```python
from build123d import *

# Parameters (mm, degrees)
BOSS_EXTRU_1_DEPTH         = 3
ESQUISSE2_W                = 10
ESQUISSE2_H                = 3
ENL_V_MAT_EXTRU_1_DEPTH    = 3
R_P_TITION_LIN_AIRE1_COUNT = 8
R_P_TITION_LIN_AIRE1_PITCH = 20
ESQUISSE4_W                = 3
ESQUISSE4_H                = 10
BOSS_EXTRU_2_DEPTH         = 3
R_P_TITION_LIN_AIRE3_COUNT = 2
R_P_TITION_LIN_AIRE3_PITCH = 20
ESQUISSE5_W                = 10
ESQUISSE5_H                = 3
ENL_V_MAT_EXTRU_3_DEPTH    = 3
R_P_TITION_LIN_AIRE4_COUNT = 4
R_P_TITION_LIN_AIRE4_PITCH = 20
ESQUISSE6_W                = 10
ESQUISSE6_H                = 3
ENL_V_MAT_EXTRU_4_DEPTH    = 3
R_P_TITION_LIN_AIRE5_COUNT = 3
R_P_TITION_LIN_AIRE5_PITCH = 20
ESQUISSE7_W                = 3
ESQUISSE7_H                = 10
ENL_V_MAT_EXTRU_5_DEPTH    = 3
R_P_TITION_LIN_AIRE6_COUNT = 3
R_P_TITION_LIN_AIRE6_PITCH = 20


with BuildPart() as part:
    # Esquisse1 → Boss.-Extru.1 (new body)
    with BuildSketch(Plane.XY):
        Polygon((163, 0), (163, -110), (113, -110), (113, -43), (0, -43), (0, 0), align=None)
    extrude(amount=BOSS_EXTRU_1_DEPTH)

    # Esquisse2 → Enlèv. mat.-Extru.1 (cut)
    with BuildSketch(Plane.XY.offset(3)):
        with Locations((5, -1.5)):
            Rectangle(ESQUISSE2_W, ESQUISSE2_H)
    enl_v_mat_extru_1 = extrude(amount=-ENL_V_MAT_EXTRU_1_DEPTH, mode=Mode.SUBTRACT)

    # Répétition linéaire1: Enlèv. mat.-Extru.1 ×8
    with Locations(*[(i * R_P_TITION_LIN_AIRE1_PITCH, 0, 0) for i in range(1, R_P_TITION_LIN_AIRE1_COUNT)]):
        add(enl_v_mat_extru_1, mode=Mode.SUBTRACT)

    # Esquisse4 → Boss.-Extru.2 (add)
    with BuildSketch(Plane.ZY):
        with Locations((1.5, -38)):
            Rectangle(ESQUISSE4_W, ESQUISSE4_H)
    boss_extru_2 = extrude(amount=BOSS_EXTRU_2_DEPTH)

    # Répétition linéaire3: Boss.-Extru.2 ×2
    with Locations(*[(0, i * R_P_TITION_LIN_AIRE3_PITCH, 0) for i in range(1, R_P_TITION_LIN_AIRE3_COUNT)]):
        add(boss_extru_2)

    # Esquisse5 → Enlèv. mat.-Extru.3 (cut)
    with BuildSketch(Plane.XY.offset(3)):
        with Locations((108, -41.5)):
            Rectangle(ESQUISSE5_W, ESQUISSE5_H)
    enl_v_mat_extru_3 = extrude(amount=-ENL_V_MAT_EXTRU_3_DEPTH, mode=Mode.SUBTRACT)

    # Répétition linéaire4: Enlèv. mat.-Extru.3 ×4
    with Locations(*[(-i * R_P_TITION_LIN_AIRE4_PITCH, 0, 0) for i in range(1, R_P_TITION_LIN_AIRE4_COUNT)]):
        add(enl_v_mat_extru_3, mode=Mode.SUBTRACT)

    # Esquisse6 → Enlèv. mat.-Extru.4 (cut)
    with BuildSketch(Plane.XY.offset(3)):
        with Locations((118, -108.5)):
            Rectangle(ESQUISSE6_W, ESQUISSE6_H)
    enl_v_mat_extru_4 = extrude(amount=-ENL_V_MAT_EXTRU_4_DEPTH, mode=Mode.SUBTRACT)

    # Répétition linéaire5: Enlèv. mat.-Extru.4 ×3
    with Locations(*[(i * R_P_TITION_LIN_AIRE5_PITCH, 0, 0) for i in range(1, R_P_TITION_LIN_AIRE5_COUNT)]):
        add(enl_v_mat_extru_4, mode=Mode.SUBTRACT)

    # Esquisse7 → Enlèv. mat.-Extru.5 (cut)
    with BuildSketch(Plane.XY.offset(3)):
        with Locations((114.5, -92)):
            Rectangle(ESQUISSE7_W, ESQUISSE7_H)
    enl_v_mat_extru_5 = extrude(amount=-ENL_V_MAT_EXTRU_5_DEPTH, mode=Mode.SUBTRACT)

    # Répétition linéaire6: Enlèv. mat.-Extru.5 ×3
    with Locations(*[(0, i * R_P_TITION_LIN_AIRE6_PITCH, 0) for i in range(1, R_P_TITION_LIN_AIRE6_COUNT)]):
        add(enl_v_mat_extru_5, mode=Mode.SUBTRACT)


solid = part.part
```
Can you work these out from the model? Positions are in its coordinate system, mm. A direction names the side the tool comes from. Coordinates: 2 decimals unless noted, no trailing zeros. Write each loop counter-clockwise with the first axis right and the second up, starting at its lowest first coordinate (ties: lowest second). Pieces come first, ordered by that corner, then holes. Notation, with made-up numbers: M 22.5,57 L 31.5,57 A37 cw 31.5,96 Z; hole C 86.25,13.5 d6. An arc over 180 degrees is marked long. Write item = value, one per line. Start each with the question number.
Q1. If we section it at A-A, the plane y = -69.5: Write out the boundary of the cut face in (x, z).
Q2. If we section it at B-B, the plane x = 67.5: Write out the boundary of the cut face in (y, z).
Q3. If I drill on L1, parallel to Y at x = 129, z = 1.15; L2, parallel to Y at x = 77, z = 1.65; L3, parallel to X at y = -12, z = 0.3, over which ranges is the centre line in solid material (lowest first)? Write a range as [from, to].
Q4. On a 3-axis mill with a long thin cutter (end or side, diameter ignored), from which of +Z, -Z, +X, -X, +Y, -Y can I reach the whole of each face in a straight line? I mean faces 1 (the face through (-1, -13, 1)), 2 (the face through (116, -52, 2)), 3 (the face through (73, -42, 2)), 4 (the face through (50, -2, 2)), 5 (the face through (113, -102, 2)). Say none if no direction works.
Q5. Thinking about a two-plate mould opening in X: for faces 6 (the face through (128, -110, 1)), 7 (the face through (113, -62, 2)), 8 (the face through (103, -42, 2)), which applies, released by +X, released by -X, zero draft, split by the parting line, or undercut?
Q6. I'm going to push flat-ended pins straight in: pin 1 (1.5 mm diameter, centred on y = -1.5, z = 1, fed in from -X); pin 2 (4 mm diameter, centred on x = 116, y = -92.5, fed in from -Z); pin 3 (1.5 mm diameter, centred on y = -29, z = 1.5, fed in from -X). Where does each tip first touch, or does it pass through?
Check sheet entries:
q1.outline = M 116,0 L 163,0 L 163,3 L 116,3 Z
q2.outline = M -40,0 L -3,0 L -3,3 L -40,3 Z
q3.L1 = [-110, -3]
q3.L2 = [-43, 0]
q3.L3 = [0, 163]
q4.face_1 = +Z, -Z, -X, +Y
q4.face_2 = +Z, -Z, -X
q4.face_3 = +Z, -Z, -Y
q4.face_4 = +Z, -Z, +Y
q4.face_5 = +Z, -Z, -X, -Y
q5.face_6 = zero draft
q5.face_7 = released by -X
q5.face_8 = undercut
q6.pin_1 = 10
q6.pin_2 = 0
q6.pin_3 = 0
